Autodesk Inventor part; units mm, degrees
ref_plane "작업 평면1" through (0, 12.5, 0) normal (0, -1, 0) x (1, 0, 0)
ref_plane "YZ Plane" through (0, 0, 0) normal (1, 0, 0) x (0, 1, 0)
ref_plane "XZ Plane" through (0, 0, 0) normal (0, 1, 0) x (-1, 0, 0)
sketch "스케치1" plane through (0, 0, 0) normal (0, 0, 1) x (1, 0, 0)
  line L0 (0, 0) -> (40, 0)
  line L1 (40, 0) -> (40, 25)
  line L2 (40, 25) -> (0, 25)
  line L3 (0, 25) -> (0, 0)
  line L4 (10, 5) -> (30, 5)
  line L5 (30, 5) -> (30, 20)
  line L6 (30, 20) -> (10, 20)
  line L7 (10, 20) -> (10, 5)
  point P0 (20, 20)
  point P1 (20, 25)
  point P2 (10, 12.5)
  point P3 (0, 12.5)
  dimension "d0" = 25
  dimension "d1" = 40
  dimension "d4" = 5
  dimension "d5" = 10
extrude "돌출1" add sketch "스케치1" along normal blind 20 contours L3 L2 L1 L0 | L7 L6 L5 L4
extrude "돌출2" cut sketch "스케치1" along normal blind 20 contours L7 L6 L5 L4
sketch "스케치2" plane through (0, 0, 0) normal (0, -1, 0) x (1, 0, 0)
  line L0 (10, 0) -> (10, 20)
  line L1 (0, 0) -> (40, 0)
  line L2 (40, 0) -> (40, 20)
  line L3 (0, 20) -> (40, 20)
  line L4 (0, 0) -> (0, 20)
  line L5 (30, 0) -> (30, 20)
  circle A0 centre (15, 10) radius 2.6
  circle A1 centre (25, 10) radius 2.6
  point P0 (10, 10)
  point P1 (20, 20)
  dimension "d11" = 5.2
  dimension "d12" = 5.2
  dimension "d13" = 10
  dimension "d14" = 5
extrude "돌출3" cut sketch "스케치2" against normal through all contours A0 | A1
ref_plane "작업 평면1" through (0, 12.5, 0) normal (0, -1, 0) x (1, 0, 0)
properties part number "다리 연결 부품-3"
Can you work these out from the model? Positions are in its coordinate system, mm. A direction names the side the tool comes from. Round coordinates to 2 decimals unless told otherwise and drop trailing zeros. Order: outer loops, then holes, each group sorted by start corner. A loop starts at its lowest first (then second) coordinate and runs counter-clockwise, first axis right, second up. Notation, with made-up numbers: (-27, 54) -> (-18, 54) arc R26 ccw to (-18, 89) -> close; hole circle Ø5 at (-5.5, -18). An arc over 180 degrees is marked (long way). Return JSON: item names as keys, results as strings. Group by question number.
1. I need wall thicknesses on line 1 (X direction, y = 7.75, z = 2.75); line 2 (Z direction, x = 15, y = 2.05); line 3 (Y direction, x = 21.5, z = 18.75). Which ranges of each line are inside material? Lowest first, please. Write a range as [from, to].
2. Which directions (+Z, -Z, +X, -X, +Y, -Y) give clear straight access to the entire face, cutting with the end or side of a thin tool? Please do faces 4 (the face through (20, 25, 10)), 5 (the face through (20, 20, 10)).
3. If we section it at B-B, the plane y = 7.5: Write out the boundary of the cut face in (x, z), then the cut area to 3 significant figures.
4. If we section it at C-C, the plane x = 15: Write out the boundary of the cut face in (y, z), then the cut area to 3 significant figures.
5. If we section it at D-D, the plane x = 29: Write out the boundary of the cut face in (y, z).
6. Will this pin go through, and if not, where does the flat tip stop? pin 1 (4.5 mm diameter, centred on x = 25, z = 10, fed in from +Y).
7. If we section it at A-A, the plane z = 10: Write out the boundary of the cut face in (x, y), then the cut area to 3 significant figures.
8. We'd pull the mould along X, two halves only. Please class faces 1 (the face through (20, 4, 20)), 2 (the face through (30, 12, 10)), 3 (the face through (0, 13, 10)): released by +X, released by -X, zero draft, split by the parting line, or undercut.
Output values:
{
 "1": {"line 1": "[0, 10], [30, 40]", "line 2": "[0, 7.4], [12.6, 20]", "line 3": "[0, 5], [20, 25]"},
 "2": {"face 4": "+Z, -Z, +X, -X, +Y", "face 5": "+Z, -Z"},
 "3": {"outline": "(0, 0) -> (10, 0) -> (10, 20) -> (0, 20) -> close; (30, 0) -> (40, 0) -> (40, 20) -> (30, 20) -> close", "area": "400 mm²"},
 "4": {"outline": "(0, 0) -> (5, 0) -> (5, 7.4) -> (0, 7.4) -> close; (0, 12.6) -> (5, 12.6) -> (5, 20) -> (0, 20) -> close; (20, 0) -> (25, 0) -> (25, 7.4) -> (20, 7.4) -> close; (20, 12.6) -> (25, 12.6) -> (25, 20) -> (20, 20) -> close", "area": "148 mm²"},
 "5": {"outline": "(0, 0) -> (5, 0) -> (5, 20) -> (0, 20) -> close; (20, 0) -> (25, 0) -> (25, 20) -> (20, 20) -> close"},
 "6": {"pin 1": "through"},
 "7": {"outline": "(0, 0) -> (12.4, 0) -> (12.4, 5) -> (10, 5) -> (10, 20) -> (12.4, 20) -> (12.4, 25) -> (0, 25) -> close; (17.6, 0) -> (22.4, 0) -> (22.4, 5) -> (17.6, 5) -> close; (17.6, 20) -> (22.4, 20) -> (22.4, 25) -> (17.6, 25) -> close; (27.6, 0) -> (40, 0) -> (40, 25) -> (27.6, 25) -> (27.6, 20) -> (30, 20) -> (30, 5) -> (27.6, 5) -> close", "area": "596 mm²"},
 "8": {"face 1": "zero draft", "face 2": "undercut", "face 3": "released by -X"}
}
